The listing builds one solid part. Answer for the finished solid, in the listing's coordinates (mm). Face numbers are marked on the shaded views. A direction names the side the tool comes from. Give positions to 0.01 mm unless a question says otherwise; leave off trailing zeros. Order: outer loops, then holes, each group sorted by start corner. A loop starts at its lowest first (then second) coordinate and runs counter-clockwise, first axis right, second up. Notation, with made-up numbers: (0.5, 82) - (13.5, 82) arc R14 ccw to (13.5, 100) - close; hole circle Ø7 at (49, 31). An arc over 180 degrees is marked (long way). Use CSV: the item, a comma, the result in double quotes.
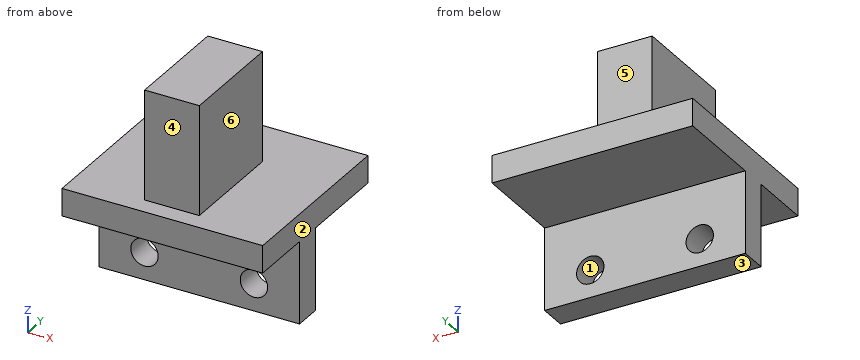
```python
from build123d import *

# Parameters (mm, degrees)
ESQUISSE1_W        = 22
ESQUISSE1_H        = 7
ESQUISSE1_R        = 1.5
BOSS_EXTRU_1_DEPTH = 3
ESQUISSE4_W        = 22
ESQUISSE4_H        = 3
BOSS_EXTRU_2_DEPTH = 5
ESQUISSE5_W        = 22
ESQUISSE5_H        = 3
BOSS_EXTRU_3_DEPTH = 10
ESQUISSE6_W        = 22
ESQUISSE6_H        = 3
BOSS_EXTRU_4_DEPTH = 7
ESQUISSE7_W        = 6
ESQUISSE7_H        = 12
BOSS_EXTRU_5_DEPTH = 12


with BuildPart() as part:
    # Esquisse1 → Boss.-Extru.1 (new body)
    with BuildSketch(Plane(origin=(0, 0, 0), x_dir=(1, 0, 0), z_dir=(0, 1, 0))):
        with Locations((2.109278351, -1.693814433)):
            Rectangle(ESQUISSE1_W, ESQUISSE1_H)
        with Locations(Location((-3.890721649, -1.193814433, 0), (0, 0, 270))):
            Circle(ESQUISSE1_R, mode=Mode.SUBTRACT)
        with Locations(Location((8.109278351, -1.193814433, 0), (0, 0, 90))):
            Circle(ESQUISSE1_R, mode=Mode.SUBTRACT)
    extrude(amount=BOSS_EXTRU_1_DEPTH)

    # Esquisse4 → Boss.-Extru.2 (add)
    with BuildSketch(Plane.XY.offset(5.193814433)):
        with Locations((2.109278351, 1.5)):
            Rectangle(ESQUISSE4_W, ESQUISSE4_H)
    extrude(amount=BOSS_EXTRU_2_DEPTH)

    # Esquisse5 → Boss.-Extru.3 (add)
    with BuildSketch(Plane(origin=(0, 3, 0), x_dir=(1, 0, 0), z_dir=(0, 1, 0))):
        with Locations((2.109278351, -8.693814433)):
            Rectangle(ESQUISSE5_W, ESQUISSE5_H)
    extrude(amount=BOSS_EXTRU_3_DEPTH)

    # Esquisse6 → Boss.-Extru.4 (add)
    with BuildSketch(Plane.XZ):
        with Locations((2.109278351, 8.693814433)):
            Rectangle(ESQUISSE6_W, ESQUISSE6_H)
    extrude(amount=BOSS_EXTRU_4_DEPTH)

    # Esquisse7 → Boss.-Extru.5 (add)
    with BuildSketch(Plane.XY.offset(10.193814433)):
        with Locations((2.009802238, 1)):
            Rectangle(ESQUISSE7_W, ESQUISSE7_H)
    extrude(amount=BOSS_EXTRU_5_DEPTH)


solid = part.part
```
Item 1: Which of the six approach directions +Z, -Z, +X, -X, +Y, -Y give full straight-line access (tool end or side, diameter ignored) to the marked faces 4, 5 and 6?
Taken from the geometry:
face 4,"+Z, +X, -X, -Y"
face 5,"+Z, +X, -X, +Y"
face 6,"+Z, +X, +Y, -Y"
Item 2: The mould has two halves that part along X. Classify the marked faces 1, 2 and 3: +X half, -X half, draft (parallel to the pull), parting line (faces both ways), or undercut.
Taken from the geometry:
face 1,"undercut"
face 2,"+X half"
face 3,"draft"
Item 3: The part is cut by section B-B (y = -4). Give the vertices of the cut face in (x, z), and give its area (3 significant figures).
Taken from the geometry:
outline,"(-8.89, 7.19) - (13.11, 7.19) - (13.11, 10.19) - (5.01, 10.19) - (5.01, 22.19) - (-0.99, 22.19) - (-0.99, 10.19) - (-8.89, 10.19) - close"
area,"138 mm^2"
Item 4: The part is cut by section A-A (x = 3.5). Give the vertices of the cut face in (y, z).
Taken from the geometry:
outline,"(-7, 7.19) - (0, 7.19) - (0, -1.81) - (3, -1.81) - (3, 7.19) - (13, 7.19) - (13, 10.19) - (7, 10.19) - (7, 22.19) - (-5, 22.19) - (-5, 10.19) - (-7, 10.19) - close"
Item 5: The part is cut by section C-C (x = 9). Give the vertices of the cut face in (y, z), and give its area (3 significant figures).
Taken from the geometry:
outline,"(-7, 7.19) - (0, 7.19) - (0, 2.4) - (3, 2.4) - (3, 7.19) - (13, 7.19) - (13, 10.19) - (-7, 10.19) - close; (0, -1.81) - (3, -1.81) - (3, -0.01) - (0, -0.01) - close"
area,"79.8 mm^2"
Item 6: Each of these flat-tipped pins is pushed along its axis until it touches: pin 1 (5 mm diameter, centred on x = 8.11, z = 1.19, fed in from +Y); pin 2 (1.8 mm diameter, centred on x = 3, z = 17.5, fed in from +Y); pin 3 (10 mm diameter, centred on x = 5.5, z = 16.5, fed in from -Y). Where does it stop, or does it pass through?
Taken from the geometry:
pin 1,"y = 3"
pin 2,"y = 7"
pin 3,"y = -5"
Item 7: Find the intervals of material crossed by line 1 along Z through (x, y) = (-5.5, -1.75); line 2 along Y through (x, z) = (2.5, 4.5); line 3 along X through (y, z) = (-1, 17.25), in increasing order.
Taken from the geometry:
line 1,"7.19 to 10.19"
line 2,"0 to 3"
line 3,"-0.99 to 5.01"
Item 8: The part is cut by section D-D (y = 2.5). Give the vertices of the cut face in (x, z), and give its area (3 significant figures).
Taken from the geometry:
outline,"(-8.89, -1.81) - (13.11, -1.81) - (13.11, 10.19) - (5.01, 10.19) - (5.01, 22.19) - (-0.99, 22.19) - (-0.99, 10.19) - (-8.89, 10.19) - close; hole circle Ø3 at (-3.89, 1.19); hole circle Ø3 at (8.11, 1.19)"
area,"322 mm^2"
